Part model, mm, in its own coordinate system. A direction names the side the tool comes from. Coordinates: 2 decimals unless noted, no trailing zeros. Loops run counter-clockwise (first coordinate to the right, second up) from the corner with the lowest first, then second, coordinate; pieces in that order, holes last. Notation, with made-up numbers: (-30.75, 17) - (-14.75, 17) arc R19 ccw to (-14.75, 26) - close; hole circle Ø8 at (35, 32). An arc over 180 degrees is marked (long way). Use a Markdown table: item, result. Add a question column.
1. Band-saw the part on B-B, the plane y = 156.5. Give the cut face in (x, z), plus the area to 3 significant figures.
2. Drop flat-ended pins along their axis: pin 1 (1.5 mm diameter, centred on x = -123.5, z = 16.5, fed in from -Y); pin 2 (6 mm diameter, centred on y = -80.5, z = 11.5, fed in from +X); pin 3 (7.5 mm diameter, centred on x = -179, z = 18, fed in from -Y). Give the stop position or say it passes through.
3. Band-saw the part on D-D, the plane x = 55. Give the cut face in (y, z), plus the area to 3 significant figures.
4. Band-saw the part on A-A, the plane y = 0. Give the cut face in (x, z), plus the area to 3 significant figures.
5. Band-saw the part on C-C, the plane x = -159.5. Give the cut face in (y, z), plus the area to 3 significant figures.
6. Pull direction X, two halves, no side cores. Call faces 1 (the cylindrical face through (-1.312, -203.196, 12.522)), 2 (the flat face through (-36.39, 80.12, 12.88)), 3 (the flat face through (-99.62, -147.15, 12.88)), 4 (the cylindrical face through (-176.63, -100.46, 12.52)): pulls with the +X half, pulls with the -X half, needs draft (parallel to the pull), parting line crosses it, or undercut.
7. Wall check: probe 1 along Y at (x, z) = (164.5, 15.5); probe 2 along X at (y, z) = (154.5, 5.5); probe 3 along X at (y, z) = (-23, 7.5). Give the ranges that are in metal, low to high. Write a range as [from, to].
8. 3-axis set-ups, long thin cutter, end or side, ignore diameter. For faces 5 (the cylindrical face through (176.63, 100.46, 12.52)), 6 (the flat face through (84.48, 24.62, 12.88)): which of +Z, -Z, +X, -X, +Y, -Y reach the whole face in a straight line?
from build123d import *

# Parameters (mm, degrees)
F0_R     = 203.2
F1_DEPTH = 25.4
F3_DEPTH = 25.401
F5_DEPTH = 25.401


with BuildPart() as f1:
    # F0 (on Top) → F1 (new body)
    with BuildSketch(Plane.XY):
        Circle(F0_R)
    extrude(amount=F1_DEPTH)

    # F2 (on face) → F3 (cut, through all)
    with BuildSketch(Plane.XY.offset(25.4)):
        with BuildLine():
            ThreePointArc((-203.2, 12.7), (-215.9, 0), (-203.2, -12.7))
            Line((-203.2, -12.7), (-152.4, -12.7))
            ThreePointArc((-152.4, -12.7), (-139.7, 0), (-152.4, 12.7))
            Line((-152.4, 12.7), (-203.2, 12.7))
        make_face()
        with BuildLine():
            Line((-87.1985226281, -125.6322715367), (-112.399890962, -169.2823219114))
            ThreePointArc((-112.399890962, -169.2823219114), (-101.6, -175.976362049), (-90.4028457059, -181.9823219114))
            Line((-90.4028457059, -181.9823219114), (-65.2014773719, -138.3322715367))
            ThreePointArc((-65.2014773719, -138.3322715367), (-69.85, -120.9837489087), (-87.1985226281, -125.6322715367))
        make_face()
        with BuildLine():
            Line((65.2014773719, -138.3322715367), (90.4028457059, -181.9823219114))
            ThreePointArc((90.4028457059, -181.9823219114), (101.6, -175.976362049), (112.399890962, -169.2823219114))
            Line((112.399890962, -169.2823219114), (87.1985226281, -125.6322715367))
            ThreePointArc((87.1985226281, -125.6322715367), (69.85, -120.9837489087), (65.2014773719, -138.3322715367))
        make_face()
        with BuildLine():
            Line((152.4, -12.7), (202.8027366679, -12.7))
            ThreePointArc((202.8027366679, -12.7), (203.1006598844, -6.353105897), (203.2, 0))
            ThreePointArc((203.2, 0), (203.1006598844, 6.353105897), (202.8027366679, 12.7))
            Line((202.8027366679, 12.7), (152.4, 12.7))
            ThreePointArc((152.4, 12.7), (139.7, 0), (152.4, -12.7))
        make_face()
        with BuildLine():
            ThreePointArc((112.399890962, 169.2823219114), (101.6, 175.976362049), (90.4028457059, 181.9823219114))
            Line((90.4028457059, 181.9823219114), (65.2014773719, 138.3322715367))
            ThreePointArc((65.2014773719, 138.3322715367), (69.85, 120.9837489087), (87.1985226281, 125.6322715367))
            Line((87.1985226281, 125.6322715367), (112.399890962, 169.2823219114))
        make_face()
        with BuildLine():
            ThreePointArc((-90.4028457059, 181.9823219114), (-101.6, 175.976362049), (-112.399890962, 169.2823219114))
            Line((-112.399890962, 169.2823219114), (-87.1985226281, 125.6322715367))
            ThreePointArc((-87.1985226281, 125.6322715367), (-69.85, 120.9837489087), (-65.2014773719, 138.3322715367))
            Line((-65.2014773719, 138.3322715367), (-90.4028457059, 181.9823219114))
        make_face()
    extrude(amount=-F3_DEPTH, mode=Mode.SUBTRACT)

    # F4 (on face) → F5 (cut, through all)
    with BuildSketch(Plane.XY.offset(25.4)):
        with BuildLine():
            ThreePointArc((76.2, 0), (75.9351262608, 6.3479602827), (75.1423464632, 12.6517891225))
            ThreePointArc((75.1423464632, 12.6517891225), (0, 76.2), (-75.1423464632, 12.6517891225))
            ThreePointArc((-75.1423464632, 12.6517891225), (-76.2, 0), (-75.1423464632, -12.6517891225))
            ThreePointArc((-75.1423464632, -12.6517891225), (0, -76.2), (75.1423464632, -12.6517891225))
            ThreePointArc((75.1423464632, -12.6517891225), (75.9351262608, -6.3479602827), (76.2, 0))
        make_face()
        with BuildLine():
            Line((-87.9951261832, 12.6517891225), (-81.5747187062, 12.6517891225))
            ThreePointArc((-81.5747187062, 12.6517891225), (-62.0869878899, 54.4032024311), (-23.2570225673, 79.2061449719))
            ThreePointArc((-23.2570225673, 79.2061449719), (-19.7040643697, 81.8658561635), (-18.7606581473, 86.2026245774))
            Line((-18.7606581473, 86.2026245774), (-25.0460243032, 85.2989253543))
            Line((-25.0460243032, 85.2989253543), (-48.0629686718, 74.7874390687))
            Line((-48.0629686718, 74.7874390687), (-67.1861371601, 58.2171192477))
            Line((-67.1861371601, 58.2171192477), (-80.866284387, 36.9303946559))
            Line((-80.866284387, 36.9303946559), (-87.9951261832, 12.6517891225))
        make_face()
        with BuildLine():
            ThreePointArc((-81.5747187062, -12.6517891225), (-82.55, 0), (-81.5747187062, 12.6517891225))
            Line((-81.5747187062, 12.6517891225), (-87.9951261832, 12.6517891225))
            Line((-87.9951261832, 12.6517891225), (-87.9951261832, -12.6517891225))
            Line((-87.9951261832, -12.6517891225), (-81.5747187062, -12.6517891225))
        make_face()
        with BuildLine():
            ThreePointArc((-75.1423464632, -12.6517891225), (-76.2, 0), (-75.1423464632, 12.6517891225))
            Line((-75.1423464632, 12.6517891225), (-81.5747187062, 12.6517891225))
            ThreePointArc((-81.5747187062, 12.6517891225), (-82.55, 0), (-81.5747187062, -12.6517891225))
            Line((-81.5747187062, -12.6517891225), (-75.1423464632, -12.6517891225))
        make_face()
        with BuildLine():
            ThreePointArc((-23.2570225673, -79.2061449719), (-62.0869878899, -54.4032024311), (-81.5747187062, -12.6517891225))
            Line((-81.5747187062, -12.6517891225), (-87.9951261832, -12.6517891225))
            Line((-87.9951261832, -12.6517891225), (-80.866284387, -36.9303946559))
            Line((-80.866284387, -36.9303946559), (-67.1861371601, -58.2171192477))
            Line((-67.1861371601, -58.2171192477), (-48.0629686718, -74.7874390687))
            Line((-48.0629686718, -74.7874390687), (-25.0460243032, -85.2989253543))
            Line((-25.0460243032, -85.2989253543), (-18.7606581473, -86.2026245774))
            ThreePointArc((-18.7606581473, -86.2026245774), (-19.7040643697, -81.8658561635), (-23.2570225673, -79.2061449719))
        make_face()
        with BuildLine():
            Line((80.866284387, -36.9303946559), (87.9951261832, -12.6517891225))
            Line((87.9951261832, -12.6517891225), (81.5747187062, -12.6517891225))
            ThreePointArc((81.5747187062, -12.6517891225), (62.0869878899, -54.4032024311), (23.2570225673, -79.2061449719))
            ThreePointArc((23.2570225673, -79.2061449719), (19.7040643697, -81.8658561635), (18.7606581473, -86.2026245774))
            Line((18.7606581473, -86.2026245774), (25.0460243032, -85.2989253543))
            Line((25.0460243032, -85.2989253543), (48.0629686718, -74.7874390687))
            Line((48.0629686718, -74.7874390687), (67.1861371601, -58.2171192477))
            Line((67.1861371601, -58.2171192477), (80.866284387, -36.9303946559))
        make_face()
        with BuildLine():
            Line((87.9951261832, -12.6517891225), (87.9951261832, 12.6517891225))
            Line((87.9951261832, 12.6517891225), (81.5747187062, 12.6517891225))
            ThreePointArc((81.5747187062, 12.6517891225), (82.55, 0), (81.5747187062, -12.6517891225))
            Line((81.5747187062, -12.6517891225), (87.9951261832, -12.6517891225))
        make_face()
        with BuildLine():
            ThreePointArc((81.5747187062, -12.6517891225), (82.55, 0), (81.5747187062, 12.6517891225))
            Line((81.5747187062, 12.6517891225), (75.1423464632, 12.6517891225))
            ThreePointArc((75.1423464632, 12.6517891225), (75.9351262608, 6.3479602827), (76.2, 0))
            ThreePointArc((76.2, 0), (75.9351262608, -6.3479602827), (75.1423464632, -12.6517891225))
            Line((75.1423464632, -12.6517891225), (81.5747187062, -12.6517891225))
        make_face()
        with BuildLine():
            Line((81.5747187062, 12.6517891225), (87.9951261832, 12.6517891225))
            Line((87.9951261832, 12.6517891225), (80.866284387, 36.9303946559))
            Line((80.866284387, 36.9303946559), (67.1861371601, 58.2171192477))
            Line((67.1861371601, 58.2171192477), (48.0629686718, 74.7874390687))
            Line((48.0629686718, 74.7874390687), (25.0460243032, 85.2989253543))
            Line((25.0460243032, 85.2989253543), (18.7606581473, 86.2026245774))
            ThreePointArc((18.7606581473, 86.2026245774), (19.7040643697, 81.8658561635), (23.2570225673, 79.2061449719))
            ThreePointArc((23.2570225673, 79.2061449719), (62.0869878899, 54.4032024311), (81.5747187062, 12.6517891225))
        make_face()
    extrude(amount=-F5_DEPTH, mode=Mode.SUBTRACT)


solid = f1.part
Geometry check:
| question | item | result |
|---|---|---|
| 1 | outline | (-129.61, 0) - (-105.02, 0) - (-105.02, 25.4) - (-129.61, 25.4) - close; (-75.69, 0) - (75.69, 0) - (75.69, 25.4) - (-75.69, 25.4) - close; (105.02, 0) - (129.61, 0) - (129.61, 25.4) - (105.02, 25.4) - close |
| 1 | area | 5,090 mm^2 |
| 2 | pin 1 | stops at y = -161.93 |
| 2 | pin 2 | stops at x = 187.84 |
| 2 | pin 3 | stops at y = -102.85 |
| 3 | outline | (-195.62, 0) - (-68.78, 0) - (-68.78, 25.4) - (-195.62, 25.4) - close; (-61.56, 0) - (-52.74, 0) - (-52.74, 25.4) - (-61.56, 25.4) - close; (52.74, 0) - (61.56, 0) - (61.56, 25.4) - (52.74, 25.4) - close; (68.78, 0) - (195.62, 0) - (195.62, 25.4) - (68.78, 25.4) - close |
| 3 | area | 6,890 mm^2 |
| 4 | outline | (-139.7, 0) - (-88, 0) - (-88, 25.4) - (-139.7, 25.4) - close; (88, 0) - (139.7, 0) - (139.7, 25.4) - (88, 25.4) - close |
| 4 | area | 2,630 mm^2 |
| 5 | outline | (-125.9, 0) - (-12.7, 0) - (-12.7, 25.4) - (-125.9, 25.4) - close; (12.7, 0) - (125.9, 0) - (125.9, 25.4) - (12.7, 25.4) - close |
| 5 | area | 5,750 mm^2 |
| 6 | face 1 | parting line crosses it |
| 6 | face 2 | undercut |
| 6 | face 3 | undercut |
| 6 | face 4 | pulls with the -X half |
| 7 | probe 1 | y = [-119.29, -12.7], [12.7, 119.29] |
| 7 | probe 2 | x = [-131.98, -103.87], [-74.54, 74.54], [103.87, 131.98] |
| 7 | probe 3 | x = [-201.89, -84.96], [-79.28, -72.65], [72.65, 79.28], [84.96, 201.89] |
| 8 | face 5 | +Z, -Z, +X, +Y |
| 8 | face 6 | +Z, -Z |
